Part model, mm, in its own coordinate system. Round coordinates to 2 decimals unless told otherwise and drop trailing zeros. Write each loop counter-clockwise with the first axis right and the second up, starting at its lowest first coordinate (ties: lowest second). Pieces come first, ordered by that corner, then holes. Notation, with made-up numbers: (66.5, 27.5) -> (105.5, 27.5) arc R25 cw to (105.5, 62.5) -> close; hole circle Ø3 at (5.5, 88.25). An arc over 180 degrees is marked (long way). Return JSON: item names as keys, results as strings. Group by question number.
(1) Mould opens along Y. For faces 1 (the flat face through (-1, 0, -1)), 2 (the flat face through (-36, 45, 1)), 3 (the cylindrical face through (-25.46, 59.99, 112.36)), 4 (the cylindrical face through (-29.644, 40.828, 112.36)) say: +Y half, -Y half, draft (parallel to the pull), parting line (faces both ways), or undercut.
(2) Drop a flat-ended pin along its axis: pin 1 Ø8 at (x, y) = (23.5, 44) entering from +Z. Give the stop position or say it passes through.
(3) Drill centre lines: L1, parallel to Z at x = -5.5, y = 58; L2, parallel to X at y = 39.5, z = 106. Where is each one in solid material? Low to high. Write a range as from..to.
(4) Saw through at C-C (z = 105). List the corners of the cut face in (x, y).
(5) Saw through at D-D (x = -26). List the corners of the cut face in (y, z).
(6) Saw through at A-A (y = 19.5). List the corners of the cut face in (x, z), plus the area to 3 significant figures.
(7) Saw through at B-B (x = 21). List the corners of the cut face in (y, z), plus the area to 3 significant figures.
from build123d import *

# Parameters (mm, degrees)
SKETCH1_W           = 72
SKETCH1_H           = 205
BOSS_EXTRUDE1_DEPTH = 90.5
SKETCH3_R           = 6.869769894
SKETCH3_R_2         = 7.145756099
BOSS_EXTRUDE2_DEPTH = 20


with BuildPart() as part:
    # Sketch1 → Boss-Extrude1 (new body)
    with BuildSketch(Plane(origin=(0, 0, 0), x_dir=(1, 0, 0), z_dir=(0, 1, 0))):
        Rectangle(SKETCH1_W, SKETCH1_H)
    extrude(amount=BOSS_EXTRUDE1_DEPTH)

    # Sketch3 → Boss-Extrude2 (add)
    with BuildSketch(Plane.XY.offset(102.5)):
        with Locations((-23.973543761, 66.695088825)):
            Circle(SKETCH3_R)
        with Locations((-23.973543761, 45.176113887)):
            Circle(SKETCH3_R_2)
    extrude(amount=BOSS_EXTRUDE2_DEPTH)


solid = part.part
Computed values:
{
 "1": {"face 1": "-Y half", "face 2": "draft", "face 3": "undercut", "face 4": "undercut"},
 "2": {"pin 1": "z = 102.5"},
 "3": {"L1": "-102.5..102.5", "L2": "-28.31..-19.63"},
 "4": {"outline": "circle Ø14.29 at (-23.97, 45.18); circle Ø13.74 at (-23.97, 66.7)"},
 "5": {"outline": "(0, -102.5) -> (90.5, -102.5) -> (90.5, 102.5) -> (73.26, 102.5) -> (73.26, 122.5) -> (60.13, 122.5) -> (60.13, 102.5) -> (52.03, 102.5) -> (52.03, 122.5) -> (38.32, 122.5) -> (38.32, 102.5) -> (0, 102.5) -> close"},
 "6": {"outline": "(-36, -102.5) -> (36, -102.5) -> (36, 102.5) -> (-36, 102.5) -> close", "area": "14,800 mm2"},
 "7": {"outline": "(0, -102.5) -> (90.5, -102.5) -> (90.5, 102.5) -> (0, 102.5) -> close", "area": "18,600 mm2"}
}
